```python
from build123d import *

# Parameters (mm, degrees)
SKETCH1_W           = 213.2
SKETCH1_H           = 208.28
SKETCH1_W_2         = 203.2
SKETCH1_H_2         = 198.28
BOSS_EXTRUDE1_DEPTH = 7
SKETCH2_W           = 203.2
SKETCH2_H           = 198.28
SKETCH2_R           = 1.5
SKETCH2_W_2         = 189.2
SKETCH2_H_2         = 184.28
BOSS_EXTRUDE2_DEPTH = 4
BOSS_EXTRUDE3_DEPTH = 57.5
BOSS_EXTRUDE4_START = -30
BOSS_EXTRUDE4_DEPTH = 64
CUT_EXTRUDE1_START  = -4
CUT_EXTRUDE1_DEPTH  = 2.5


with BuildPart() as part:
    # Sketch1 → Boss-Extrude1 (new body)
    with BuildSketch(Plane.XY):
        Rectangle(SKETCH1_W, SKETCH1_H)
        Rectangle(SKETCH1_W_2, SKETCH1_H_2, mode=Mode.SUBTRACT)
    extrude(amount=BOSS_EXTRUDE1_DEPTH)

    # Sketch2 → Boss-Extrude2 (add)
    with BuildSketch(Plane.XY):
        Rectangle(SKETCH2_W, SKETCH2_H)
        with Locations((0, 95.64)):
            Circle(SKETCH2_R, mode=Mode.SUBTRACT)
        with Locations((-98.1, 0)):
            Circle(SKETCH2_R, mode=Mode.SUBTRACT)
        with Locations(Location((98.1, 0, 0), (0, 0, 180))):
            Circle(SKETCH2_R, mode=Mode.SUBTRACT)
        Rectangle(SKETCH2_W_2, SKETCH2_H_2, mode=Mode.SUBTRACT)
    extrude(amount=BOSS_EXTRUDE2_DEPTH)

    # Sketch3 → Boss-Extrude3 (add)
    with BuildSketch(Plane.XY.offset(7)):
        Polygon((-106.6, 104.14), (-106.6, -104.14), (-101.6, -104.14), (-101.6, -99.14), (-101.6, 99.14), (-101.6, 104.14), align=None)
        Polygon((101.6, -99.14), (101.6, -104.14), (106.6, -104.14), (106.6, 104.14), (101.6, 104.14), (101.6, 99.14), align=None)
    extrude(amount=BOSS_EXTRUDE3_DEPTH)

    # Sketch4 → Boss-Extrude4 (add)
    with BuildSketch(Plane(origin=(0, 104.14, 0), x_dir=(1, 0, 0), z_dir=(0, 1, 0)).offset(BOSS_EXTRUDE4_START)):
        with BuildLine():
            Line((-101.6, -59.8), (-101.6, -64.5))
            ThreePointArc((-101.6, -64.5), (-99.952936105, -62.15), (-101.6, -59.8))
        make_face()
        with BuildLine():
            Line((101.6, -59.8), (101.6, -64.5))
            ThreePointArc((101.6, -64.5), (99.952936105, -62.15), (101.6, -59.8))
        make_face()
        with BuildLine():
            Line((-101.6, -50.1), (-101.6, -54.8))
            ThreePointArc((-101.6, -54.8), (-99.952936105, -52.45), (-101.6, -50.1))
        make_face()
        with BuildLine():
            Line((101.6, -50.1), (101.6, -54.8))
            ThreePointArc((101.6, -54.8), (99.952936105, -52.45), (101.6, -50.1))
        make_face()
    extrude(amount=-BOSS_EXTRUDE4_DEPTH)

    # Sketch5 → Cut-Extrude1 (cut)
    with BuildSketch(Plane.XY.offset(4).offset(CUT_EXTRUDE1_START)):
        Polygon((-95.325, -1.602146997), (-95.325, 1.602146997), (-98.1, 3.204293994), (-100.875, 1.602146997), (-100.875, -1.602146997), (-98.1, -3.204293994), align=None)
        Polygon((98.1, -3.204293994), (95.325, -1.602146997), (95.325, 1.602146997), (98.1, 3.204293994), (100.875, 1.602146997), (100.875, -1.602146997), align=None)
        Polygon((1.602146997, 92.865), (3.204293994, 95.64), (1.602146997, 98.415), (-1.602146997, 98.415), (-3.204293994, 95.64), (-1.602146997, 92.865), align=None)
    extrude(amount=CUT_EXTRUDE1_DEPTH, mode=Mode.SUBTRACT)


solid = part.part
```
Geometry check sheet. Reference: the model listing, model coordinates, mm. A direction names the side the tool comes from. Coordinates: 2 decimals unless noted, no trailing zeros. Loops run counter-clockwise (first coordinate to the right, second up) from the corner with the lowest first, then second, coordinate; pieces in that order, holes last.
Item 1: Thickness scan on line 1 (Y direction, x = 0, z = 3.6); line 2 (Y direction, x = -98, z = 3); line 3 (X direction, y = 59, z = 58). Record the ranges inside material, lowest first.
Item 2: Release check for a two-part mould opening along Z. For faces 1 (the face through (-99.953, 42.588, 52.493)), 2 (the face through (-95, 16, 0)), 3 (the face through (-104, 1, 64.5)) record: released by +Z, released by -Z, zero draft, split by the parting line, or undercut.
Item 3: Sectioned sample at A-A, the plane y = -86.5. Record the boundary of the cut face in (x, z).
Item 4: Sectioned sample at D-D, the plane y = 25.5. Record the boundary of the cut face in (x, z), then the cut area to 3 significant figures.
Item 5: Sectioned sample at C-C, the plane x = 61.5. Record the boundary of the cut face in (y, z).
Item 6: Sectioned sample at B-B, the plane z = 12. Record the boundary of the cut face in (x, y).
Item 7: Access from +Z, -Z, +X, -X, +Y, -Y to the whole of each face (thin tool, end or side, straight path). Record for faces 4 (the face through (-1, -102, 7)), 5 (the face through (99.953, 42.588, 62.193)), 6 (the face through (101.6, 1, 34)).
Item 8: Go/stop test with flat-tipped pins: pin 1 Ø4.5 at (x, y) = (1, 95) entering from -Z; pin 2 Ø0.5 at (x, z) = (-101, 52.5) entering from +Y; pin 3 Ø1.7 at (x, y) = (-99, 1) entering from -Z. Record where each tip stops, or that it passes through.
Check result:
1. line 1: y = -104.14 to -92.14, 92.14 to 94.14, 97.14 to 104.14
1. line 2: y = -104.14 to -1.5, 1.5 to 104.14
1. line 3: x = -106.6 to -101.6, 101.6 to 106.6
2. face 1: undercut
2. face 2: released by -Z
2. face 3: released by +Z
3. outline: (-106.6, 0) - (-94.6, 0) - (-94.6, 4) - (-101.6, 4) - (-101.6, 64.5) - (-106.6, 64.5) - close; (94.6, 0) - (106.6, 0) - (106.6, 64.5) - (101.6, 64.5) - (101.6, 4) - (94.6, 4) - close
4. outline: (-106.6, 0) - (-94.6, 0) - (-94.6, 4) - (-101.6, 4) - (-101.6, 50.1) arc R2.5 ccw to (-101.6, 54.8) - (-101.6, 59.8) arc R2.5 ccw to (-101.6, 64.5) - (-106.6, 64.5) - close; (94.6, 0) - (106.6, 0) - (106.6, 64.5) - (101.6, 64.5) arc R2.5 ccw to (101.6, 59.8) - (101.6, 54.8) arc R2.5 ccw to (101.6, 50.1) - (101.6, 4) - (94.6, 4) - close
4. area: 724 mm2
5. outline: (-104.14, 0) - (-92.14, 0) - (-92.14, 4) - (-99.14, 4) - (-99.14, 7) - (-104.14, 7) - close; (92.14, 0) - (104.14, 0) - (104.14, 7) - (99.14, 7) - (99.14, 4) - (92.14, 4) - close
6. outline: (-106.6, -104.14) - (-101.6, -104.14) - (-101.6, 104.14) - (-106.6, 104.14) - close; (101.6, -104.14) - (106.6, -104.14) - (106.6, 104.14) - (101.6, 104.14) - close
7. face 4: +Z, +Y, -Y
7. face 5: +Y, -Y
7. face 6: none
8. pin 1: stops at z = 0
8. pin 2: stops at y = 74.14
8. pin 3: stops at z = 2.5
